from build123d import *

# Parameters (mm, degrees)
F1_DEPTH = 40
F3_DEPTH = 30
F5_DEPTH = 30


with BuildPart() as f1:
    # F0 (on Front) → F1 (new body)
    with BuildSketch(Plane.XZ):
        with BuildLine():
            Line((-57.0404038358, 50), (-31.5845597131, 24.5441558773))
            ThreePointArc((-31.5845597131, 24.5441558773), (17.5817201222, -35.9288619016), (0, 40))
            Line((0, 40), (42.9595961642, 40))
            Line((42.9595961642, 40), (42.9595961642, 50))
            Line((42.9595961642, 50), (-57.0404038358, 50))
        make_face()
    extrude(amount=F1_DEPTH)

    # F2 (on face) → F3 (join)
    with BuildSketch(Plane.XZ.offset(40)):
        with BuildLine():
            ThreePointArc((-31.5845597131, 24.5441558773), (-17.5817201222, 35.9288619016), (0, 40))
            Line((0, 40), (42.9595961642, 40))
            Line((42.9595961642, 40), (42.9595961642, 50))
            Line((42.9595961642, 50), (-57.0404038358, 50))
            Line((-57.0404038358, 50), (-31.5845597131, 24.5441558773))
        make_face()
    extrude(amount=F3_DEPTH)

    # F4 (on face) → F5 (join)
    with BuildSketch(Plane(origin=(0, 0, 0), x_dir=(-1, 0, 0), z_dir=(0, 1, 0))):
        with BuildLine():
            ThreePointArc((0, 40), (17.5817201222, 35.9288619016), (31.5845597131, 24.5441558773))
            Line((31.5845597131, 24.5441558773), (57.0404038358, 50))
            Line((57.0404038358, 50), (-42.9595961642, 50))
            Line((-42.9595961642, 50), (-42.9595961642, 40))
            Line((-42.9595961642, 40), (0, 40))
        make_face()
    extrude(amount=F5_DEPTH)


solid = f1.part
Verification items for the finished model (mm, model axes). A direction names the side the tool comes from. Give positions to 0.01 mm unless a question says otherwise; leave off trailing zeros. Order: outer loops, then holes, each group sorted by start corner. A loop starts at its lowest first (then second) coordinate and runs counter-clockwise, first axis right, second up. Notation, with made-up numbers: (2, 15) -> (12, 15) arc R10 ccw to (12, 29) -> close; hole circle Ø11 at (84, -2.5). An arc over 180 degrees is marked (long way). Answer as CSV lines item,"result".
Q1. Access from +Z, -Z, +X, -X, +Y, -Y to the whole of each face (thin tool, end or side, straight path). Record for faces 1 (the flat face through (-8, -70, 43)), 2 (the cylindrical face through (-17.35, 14.79, 36.04)), 3 (the flat face through (-1, -40, 1)).
Solutions:
face 1,"+Z, -Z, +X, -X, -Y"
face 2,"-Z, +X, +Y"
face 3,"-Z, +X, -Y"
Q2. Sectioned sample at A-A on x = 33.5. Record the cut outline in (y, z).
Solutions:
outline,"(-70, 40) -> (30, 40) -> (30, 50) -> (-70, 50) -> close; (-40, -21.86) -> (0, -21.86) -> (0, 21.86) -> (-40, 21.86) -> close"
Q3. Sectioned sample at C-C on x = -16.5. Record the cut outline in (y, z).
Solutions:
outline,"(-70, 36.44) -> (-40, 36.44) -> (-40, -36.44) -> (0, -36.44) -> (0, 36.44) -> (30, 36.44) -> (30, 50) -> (-70, 50) -> close"
Q4. Depth check by flat-ended pin: pin 1 (1 mm diameter, centred on x = -36.5, z = 3.5, fed in from -Y); pin 2 (1 mm diameter, centred on x = 7.5, z = -1.5, fed in from +Y); pin 3 (21.5 mm diameter, centred on x = 32, y = -31.5, fed in from -Z). Enter the tip coordinate at first touch or a pass-through.
Solutions:
pin 1,"stops at y = -40"
pin 2,"stops at y = 0"
pin 3,"stops at z = -33.89"
Q5. Scan lines: probe 1 along Z at (x, y) = (35.5, -55); probe 2 along Y at (x, z) = (16.5, 26); probe 3 along Z at (x, y) = (37, -36.5). Record each from-to range of solid material in increasing order.
Solutions:
probe 1,"z = 40 to 50"
probe 2,"y = -40 to 0"
probe 3,"z = -15.2 to 15.2, 40 to 50"
Q6. Release check for a two-part mould opening along Z. For faces 4 (the cylindrical face through (16.218, -19.72, -36.565)), 5 (the flat face through (-8, -21, 50)), 6 (the flat face through (-1, 0, 1)) record: +Z half, -Z half, draft (parallel to the pull), parting line (faces both ways), or undercut.
Solutions:
face 4,"undercut"
face 5,"+Z half"
face 6,"draft"
Q7. Sectioned sample at B-B on y = 12.5. Record the cut outline in (x, z), plus the area to 3 significant figures.
Solutions:
outline,"(-57.04, 50) -> (-31.58, 24.54) arc R40 cw to (0, 40) -> (42.96, 40) -> (42.96, 50) -> close"
area,"1,220 mm²"
Q8. Sectioned sample at D-D on z = 0. Record the cut outline in (x, y), plus the area to 3 significant figures.
Solutions:
outline,"(-40, -40) -> (40, -40) -> (40, 0) -> (-40, 0) -> close"
area,"3,200 mm²"
